Here's how the part is built. I have some questions about the finished solid (model axes, mm). Face numbers are marked on the shaded views. A direction names the side the tool comes from. Give positions to 0.01 mm unless a question says otherwise; leave off trailing zeros. Loops run counter-clockwise (first coordinate to the right, second up) from the corner with the lowest first, then second, coordinate; pieces in that order, holes last. Notation, with made-up numbers: (47.25, 71) - (66.25, 71) arc R17 ccw to (66.25, 90) - close; hole circle Ø9 at (34, 45). An arc over 180 degrees is marked (long way). Use one line per item in the form item = value.
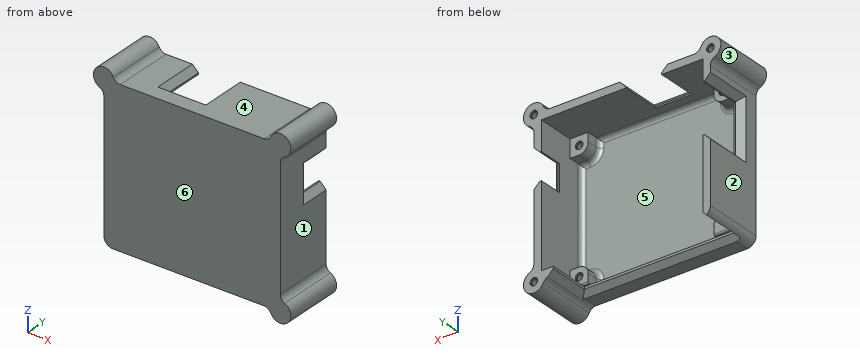
from build123d import *

# Parameters (mm, degrees)
SKETCH1_W               = 118
SKETCH1_H               = 103
SKETCH1_W_2             = 108
SKETCH1_H_2             = 93
SKETCH1_W_3             = 106
SKETCH1_H_3             = 91
BOSS_EXTRUDE1_DEPTH     = 5
SKETCH2_W               = 118
SKETCH2_H               = 103
SKETCH2_W_2             = 108
SKETCH2_H_2             = 93
BOSS_EXTRUDE2_DEPTH     = 35.6
SKETCH3_W               = 12
SKETCH3_H               = 12
BOSS_EXTRUDE3_DEPTH     = 10
MIRROR5_COPY_1_SKETCH_W = 12
MIRROR5_COPY_1_SKETCH_H = 12
MIRROR5_COPY_1_DEPTH    = 10
SKETCH4_R               = 2
CUT_EXTRUDE1_DEPTH      = 6
SKETCH4_3_R             = 2.525
CUT_EXTRUDE2_DEPTH      = 1
SKETCH6_W               = 100
SKETCH6_H               = 27.6
CUT_EXTRUDE3_DEPTH      = 122.381052887
SKETCH7_W               = 33
SKETCH7_H               = 27.6
CUT_EXTRUDE4_DEPTH      = 131.650717564
SKETCH8_W               = 24
SKETCH8_H               = 26.6
CUT_EXTRUDE5_DEPTH      = 122.381052887
CHAMFER1_SIZE           = 3.5
SKETCH10_W              = 18
SKETCH10_H              = 16
CUT_EXTRUDE7_DEPTH      = 131.650717564
SKETCH11_R              = 7
BOSS_EXTRUDE4_DEPTH     = 40.6
FILLET1_R               = 6
CHAMFER2_SIZE           = 4
CHAMFER3_SIZE           = 4
FILLET2_R               = 3
CHAMFER4_SIZE           = 4
FILLET7_R               = 5
FILLET8_R               = 1
FILLET9_R               = 6
SKETCH12_R              = 2
CUT_EXTRUDE9_DEPTH      = 10
SKETCH12_3_R            = 2.55
CUT_EXTRUDE10_DEPTH     = 1


with BuildPart() as part:
    # Sketch1 → Boss-Extrude1 (new body)
    # profile 1 of 3: a face of its own
    with BuildSketch(Plane(origin=(0, 0, 0), x_dir=(1, 0, 0), z_dir=(0, 1, 0))):
        Rectangle(SKETCH1_W, SKETCH1_H)
        Rectangle(SKETCH1_W_2, SKETCH1_H_2, mode=Mode.SUBTRACT)
    # profile 2 of 3: a face of its own
    with BuildSketch(Plane(origin=(0, 0, 0), x_dir=(1, 0, 0), z_dir=(0, 1, 0))):
        Rectangle(SKETCH1_W_2, SKETCH1_H_2)
        Rectangle(SKETCH1_W_3, SKETCH1_H_3, mode=Mode.SUBTRACT)
    # profile 3 of 3: a face of its own
    with BuildSketch(Plane(origin=(0, 0, 0), x_dir=(1, 0, 0), z_dir=(0, 1, 0))):
        Rectangle(SKETCH1_W_3, SKETCH1_H_3)
    extrude(amount=BOSS_EXTRUDE1_DEPTH)

    # Sketch2 → Boss-Extrude2 (add)
    with BuildSketch(Plane(origin=(0, 5, 0), x_dir=(1, 0, 0), z_dir=(0, 1, 0))):
        Rectangle(SKETCH2_W, SKETCH2_H)
        Rectangle(SKETCH2_W_2, SKETCH2_H_2, mode=Mode.SUBTRACT)
    extrude(amount=BOSS_EXTRUDE2_DEPTH)

    # Sketch3 → Boss-Extrude3 (add)
    with BuildSketch(Plane(origin=(0, 5, 0), x_dir=(1, 0, 0), z_dir=(0, 1, 0))):
        with Locations((48, -40.5)):
            Rectangle(SKETCH3_W, SKETCH3_H)
    boss_extrude3 = extrude(amount=BOSS_EXTRUDE3_DEPTH)

    # Mirror4: Boss-Extrude3 across plane
    add(boss_extrude3.mirror(Plane(origin=(0, 0, 0), x_dir=(0, 0, 1), z_dir=(1, 0, 0))))

    # Mirror5: Boss-Extrude3 across plane
    add(boss_extrude3.mirror(Plane.XY))

    # Mirror5 copy 1 sketch → Mirror5 copy 1 (add)
    with BuildSketch(Plane(origin=(0, 5, 0), x_dir=(-1, 0, 0), z_dir=(0, 1, 0))):
        with Locations((48, -40.5)):
            Rectangle(MIRROR5_COPY_1_SKETCH_W, MIRROR5_COPY_1_SKETCH_H)
    extrude(amount=MIRROR5_COPY_1_DEPTH)

    # Sketch4 → Cut-Extrude1 (cut)
    with BuildSketch(Plane(origin=(0, 15, 0), x_dir=(1, 0, 0), z_dir=(0, 1, 0))):
        with Locations(Location((48, -40.5, 0), (0, 0, 270))):
            Circle(SKETCH4_R)
    cut_extrude1 = extrude(amount=-CUT_EXTRUDE1_DEPTH, mode=Mode.SUBTRACT)

    # Sketch4<3> → Cut-Extrude2 (cut)
    with BuildSketch(Plane(origin=(0, 15, 0), x_dir=(1, 0, 0), z_dir=(0, 1, 0))):
        with Locations(Location((48, -40.5, 0), (0, 0, 270))):
            Circle(SKETCH4_3_R)
    cut_extrude2 = extrude(amount=-CUT_EXTRUDE2_DEPTH, mode=Mode.SUBTRACT)

    # Mirror2: Boss-Extrude3, Cut-Extrude1, Cut-Extrude2 across plane
    add(boss_extrude3.mirror(Plane.XY))
    add(cut_extrude1.mirror(Plane.XY), mode=Mode.SUBTRACT)
    add(cut_extrude2.mirror(Plane.XY), mode=Mode.SUBTRACT)

    # Mirror2 at the second plane: Boss-Extrude3, Cut-Extrude1, Cut-Extrude2 across plane
    add(boss_extrude3.mirror(Plane(origin=(0, 0, 0), x_dir=(0, 0, 1), z_dir=(1, 0, 0))))
    add(cut_extrude1.mirror(Plane(origin=(0, 0, 0), x_dir=(0, 0, 1), z_dir=(1, 0, 0))), mode=Mode.SUBTRACT)
    add(cut_extrude2.mirror(Plane(origin=(0, 0, 0), x_dir=(0, 0, 1), z_dir=(1, 0, 0))), mode=Mode.SUBTRACT)

    # Sketch6 → Cut-Extrude3 (cut, through all)
    with BuildSketch(Plane.XY.offset(-46.5)):
        with Locations((-4, 26.8)):
            Rectangle(SKETCH6_W, SKETCH6_H)
    extrude(amount=-CUT_EXTRUDE3_DEPTH, mode=Mode.SUBTRACT)

    # Sketch7 → Cut-Extrude4 (cut, through all)
    with BuildSketch(Plane(origin=(-54, 0, 0), x_dir=(0, 0, -1), z_dir=(1, 0, 0))):
        with Locations((-16, 26.8)):
            Rectangle(SKETCH7_W, SKETCH7_H)
    extrude(amount=-CUT_EXTRUDE4_DEPTH, mode=Mode.SUBTRACT)

    # Sketch8 → Cut-Extrude5 (cut, through all)
    with BuildSketch(Plane(origin=(0, 0, 46.5), x_dir=(-1, 0, 0), z_dir=(0, 0, -1))):
        with Locations((14.4, 27.3)):
            Rectangle(SKETCH8_W, SKETCH8_H)
    extrude(amount=-CUT_EXTRUDE5_DEPTH, mode=Mode.SUBTRACT)

    # Chamfer1
    chamfer1_edges = [part.edges().sort_by_distance(p)[0] for p in [
        (-54, 26.8, -51.5),
        (46, 26.8, -51.5),
        (-4, 13, -51.5),
    ]]
    chamfer(chamfer1_edges, length=CHAMFER1_SIZE)

    # Sketch10 → Cut-Extrude7 (cut, through all)
    with BuildSketch(Plane.ZY.offset(-54)):
        with Locations((18, 32.6)):
            Rectangle(SKETCH10_W, SKETCH10_H)
    extrude(amount=-CUT_EXTRUDE7_DEPTH, mode=Mode.SUBTRACT)

    # Sketch11 → Boss-Extrude4 (add)
    with BuildSketch(Plane(origin=(0, 0, 0), x_dir=(1, 0, 0), z_dir=(0, 1, 0))):
        with Locations((59, -51.5)):
            Circle(SKETCH11_R)
        with Locations((59, 51.5)):
            Circle(SKETCH11_R)
        with Locations((-59, -51.5)):
            Circle(SKETCH11_R)
    extrude(amount=BOSS_EXTRUDE4_DEPTH)

    # Fillet1
    fillet1_edges = [part.edges().sort_by_distance(p)[0] for p in [
        (42, 10, 34.5),
        (-42, 10, 34.5),
        (-42, 10, -34.5),
        (42, 10, -34.5),
    ]]
    fillet(fillet1_edges, radius=FILLET1_R)

    # Chamfer2
    chamfer2_edges = [part.edges().sort_by_distance(p)[0] for p in [
        (-59, 26.8, 32.5),
        (-59, 26.8, -0.5),
        (-59, 13, 16),
    ]]
    chamfer(chamfer2_edges, length=CHAMFER2_SIZE)

    # Chamfer3
    chamfer3_edges = [part.edges().sort_by_distance(p)[0] for p in [
        (-26.4, 27.3, 51.5),
        (-14.4, 14, 51.5),
        (-2.4, 27.3, 51.5),
    ]]
    chamfer(chamfer3_edges, length=CHAMFER3_SIZE)

    # Fillet2
    fillet2_edges = [part.edges().sort_by_distance(p)[0] for p in [
        (-42, 5, 43.5),
        (-42, 5, -43.5),
        (42, 5, -43.5),
        (42, 5, 43.5),
        (-43.757359313, 5, 36.257359313),
        (-43.757359313, 5, -36.257359313),
        (43.757359313, 5, -36.257359313),
        (43.757359313, 5, 36.257359313),
        (54, 5, 0),
        (51, 5, 34.5),
        (0, 5, 46.5),
        (-51, 5, 34.5),
        (-54, 5, 0),
        (-51, 5, -34.5),
        (0, 5, -46.5),
        (51, 5, -34.5),
    ]]
    fillet(fillet2_edges, radius=FILLET2_R)

    # Chamfer4
    chamfer4_edges = [part.edges().sort_by_distance(p)[0] for p in [
        (59, 32.6, 9),
        (59, 32.6, 27),
        (59, 24.6, 18),
    ]]
    chamfer(chamfer4_edges, length=CHAMFER4_SIZE)

    # Fillet7
    fillet7_edges = [part.edges().sort_by_distance(p)[0] for p in [
        (52, 20.3, -51.5),
        (59, 20.3, -44.5),
        (59, 20.3, 44.5),
        (52, 20.3, 51.5),
        (-52, 20.3, 51.5),
        (-59, 20.3, 44.5),
    ]]
    fillet(fillet7_edges, radius=FILLET7_R)

    # Fillet8
    fillet8_edges = [part.edges().sort_by_distance(p)[0] for p in [
        (-48, 15, -46.5),
        (44, 15, -46.5),
    ]]
    fillet(fillet8_edges, radius=FILLET8_R)

    # Fillet9
    fillet9_edges = [part.edges().sort_by_distance(p)[0] for p in [
        (-59, 20.3, -51.5),
    ]]
    fillet(fillet9_edges, radius=FILLET9_R)

    # Sketch12 → Cut-Extrude9 (cut)
    with BuildSketch(Plane(origin=(0, 40.6, 0), x_dir=(1, 0, 0), z_dir=(0, 1, 0))):
        with Locations(Location((59, -51.5, 0), (0, 0, 270))):
            Circle(SKETCH12_R)
    cut_extrude9 = extrude(amount=-CUT_EXTRUDE9_DEPTH, mode=Mode.SUBTRACT)

    # Sketch12<3> → Cut-Extrude10 (cut)
    with BuildSketch(Plane(origin=(0, 40.6, 0), x_dir=(1, 0, 0), z_dir=(0, 1, 0))):
        with Locations(Location((59, -51.5, 0), (0, 0, 270))):
            Circle(SKETCH12_3_R)
    cut_extrude10 = extrude(amount=-CUT_EXTRUDE10_DEPTH, mode=Mode.SUBTRACT)

    # Mirror6: Cut-Extrude9, Cut-Extrude10 across plane
    add(cut_extrude9.mirror(Plane(origin=(0, 0, 0), x_dir=(0, 0, 1), z_dir=(1, 0, 0))), mode=Mode.SUBTRACT)
    add(cut_extrude10.mirror(Plane(origin=(0, 0, 0), x_dir=(0, 0, 1), z_dir=(1, 0, 0))), mode=Mode.SUBTRACT)

    # Mirror6 at the second plane: Cut-Extrude9, Cut-Extrude10 across plane
    add(cut_extrude9.mirror(Plane.XY), mode=Mode.SUBTRACT)
    add(cut_extrude10.mirror(Plane.XY), mode=Mode.SUBTRACT)


solid = part.part
(1) If we section it at A-A (y = 18.5): Give the number of separate pieces and of enclosed holes in the cut face, plus the area to 3 significant figures.
Geometry says:
separate_pieces = 3
enclosed_holes = 0
area = 1,640 mm²
(2) If we section it at D-D (x = 10): List the corners of the cut face in (y, z) for me, plus the area to 3 significant figures.
Geometry says:
outline = (0, -51.5) - (9.5, -51.5) - (13, -48) - (13, -46.5) - (8, -46.5) arc R3 cw to (5, -43.5) - (5, 43.5) arc R3 cw to (8, 46.5) - (40.6, 46.5) - (40.6, 51.5) - (0, 51.5) - close
area = 731 mm²
(3) Thinking about a two-plate mould opening in Z: for the marked faces 1, 2, 3 and 4, which applies, pulls with the +Z half, pulls with the -Z half, needs draft (parallel to the pull), parting line crosses it, or undercut?
Geometry says:
face_1 = undercut
face_2 = needs draft
face_3 = parting line crosses it
face_4 = pulls with the +Z half
(4) For the marked faces 5 and 6, which set-ups out of +Z, -Z, +X, -X, +Y, -Y let a thin tool reach every point of the face, with its end or its side?
Geometry says:
face_5 = +Y
face_6 = +Z, -Z, +X, -X, -Y
(5) If we section it at B-B (z = 17): List the corners of the cut face in (x, y) for me.
Geometry says:
outline = (-59, 0) - (59, 0) - (59, 20.6) - (55, 24.6) - (54, 24.6) - (54, 8) arc R3 cw to (51, 5) - (-51, 5) arc R3 cw to (-54, 8) - (-54, 13) - (-55, 13) - (-59, 9) - close
(6) For P1, Ø8, axis at x = 32.5, y = 22, coming from the -Z side; P2, Ø6, axis at x = 45.5, z = -40.5, coming from the +Y side; P3, Ø3, axis at y = 31.5, z = -7, coming from the -X side; P4, Ø3, axis at x = -8.5, y = 16, coming from the -Z side, each with a flat end and sliding along its axis, tell me the tip position at first contact or that it passes through.
Geometry says:
P1 = 46.5
P2 = 15
P3 = -59
P4 = through
(7) If we section it at C-C (y = 3.5): List the corners of the cut face in (x, z) for me, plus the area to 3 significant figures.
Geometry says:
outline = (-61.92, 45.14) arc R5 cw to (-59, 40.59) - (-59, -45.5) arc R6 ccw to (-53, -51.5) - (48.09, -51.5) arc R5 cw to (52.64, -54.42) arc R7 ccw (long way) to (61.92, -45.14) arc R5 cw to (59, -40.59) - (59, 40.59) arc R5 cw to (61.92, 45.14) arc R7 ccw (long way) to (52.64, 54.42) arc R5 cw to (48.09, 51.5) - (-48.09, 51.5) arc R5 cw to (-52.64, 54.42) arc R7 ccw (long way) to start
area = 12,500 mm²
(8) If I drill on probe 1 along X at (y, z) = (14.6, 40.5) (3 decimals); probe 2 along X at (y, z) = (26, -36.5); probe 3 along X at (y, z) = (40.3, -51.5), over which ranges is the centre line in solid material (lowest first)?
Geometry says:
probe_1 = -59 to -50.525, -45.475 to -42, 42 to 45.475, 50.525 to 59
probe_2 = -59 to -54, 54 to 59
probe_3 = 49.5 to 56.45, 61.55 to 66
